from build123d import *

# Parameters (mm, degrees)
BOSS_EXTRUDE1_DEPTH      = 520.7
BOSS_EXTRUDE1_DEPTH_BACK = 520.7
SKETCH1_W                = 38.1
SKETCH1_H                = 25.4
SKETCH1_W_2              = 31.75
SKETCH1_H_2              = 19.05
SKETCH2_R                = 2.38125
CUT_EXTRUDE1_DEPTH       = 520.7
SKETCH3_R                = 2.38125
CUT_EXTRUDE2_DEPTH       = 100


with BuildPart() as part:
    # Sketch1 → Boss-Extrude1 (new, two sides: drawn at the far end of the back side and taken through both)
    with BuildSketch(Plane.XY.offset(-BOSS_EXTRUDE1_DEPTH_BACK)):
        Rectangle(SKETCH1_W, SKETCH1_H)
        Rectangle(SKETCH1_W_2, SKETCH1_H_2, mode=Mode.SUBTRACT)
    extrude(amount=BOSS_EXTRUDE1_DEPTH + BOSS_EXTRUDE1_DEPTH_BACK)

    # Sketch2 → Cut-Extrude1 (cut)
    with BuildSketch(Plane(origin=(0, 12.7, 0), x_dir=(1, 0, 0), z_dir=(0, 1, 0))):
        with Locations(Location((0, -384.81, 0), (0, 0, 180))):
            Circle(SKETCH2_R)
        with Locations(Location((0, -505.46, 0), (0, 0, 180))):
            Circle(SKETCH2_R)
    extrude(amount=-CUT_EXTRUDE1_DEPTH, mode=Mode.SUBTRACT)

    # Sketch3 → Cut-Extrude2 (cut)
    with BuildSketch(Plane(origin=(0, 12.7, 0), x_dir=(1, 0, 0), z_dir=(0, 1, 0))):
        with Locations(Location((0, 506.4125, 0), (0, 0, 180))):
            Circle(SKETCH3_R)
        with Locations(Location((0, 466.725, 0), (0, 0, 180))):
            Circle(SKETCH3_R)
    extrude(amount=-CUT_EXTRUDE2_DEPTH, mode=Mode.SUBTRACT)


solid = part.part
Source: CAD feature listing. Evaluate the final solid. Frame: model axes, mm. A direction names the side the tool comes from. Give positions to 0.01 mm unless a question says otherwise; leave off trailing zeros. Write each loop counter-clockwise with the first axis right and the second up, starting at its lowest first coordinate (ties: lowest second). Pieces come first, ordered by that corner, then holes. Notation, with made-up numbers: M -10,11 L -6,11 A8 cw -6,15 Z; hole C 51,68 d4. An arc over 180 degrees is marked long. Answer as a JSON object with one key per item and string values.
Q1. Cut plane A-A, the plane x = -8.5. Return the cut outline in (y, z) (3 decimals).
Geometry check:
{"outline": "M -12.7,-520.7 L -9.525,-520.7 L -9.525,520.7 L -12.7,520.7 Z; M 9.525,-520.7 L 12.7,-520.7 L 12.7,520.7 L 9.525,520.7 Z"}
Q2. Ray query, line 1 along Z through (x, y) = (0, 11.5); line 2 along X through (y, z) = (-1, -285) (3 decimals); line 3 along X through (y, z) = (-12, 505.46). Return the intervals inside material, ascending.
Geometry check:
{"line 1": "z = -520.7 to -508.79, -504.03 to -469.11, -464.34 to 382.43, 387.19 to 503.08, 507.84 to 520.7", "line 2": "x = -19.05 to -15.875, 15.875 to 19.05", "line 3": "x = -19.05 to -2.38, 2.38 to 19.05"}
Q3. Mould query, pull axis Y, two halves, no side actions, for faces 3 (the face through (0, 12.7, -7)), 4 (the face through (0, -9.525, -7)), 5 (the face through (0, -11, 520.7)). Classes: +Y half, -Y half, draft (parallel to the pull), parting line (faces both ways), or undercut.
Geometry check:
{"face 3": "+Y half", "face 4": "undercut", "face 5": "draft"}
Q4. Cut plane B-B, the plane z = -267.5. Return the cut outline in (x, y) (3 decimals), then the cut area to 3 significant figures.
Geometry check:
{"outline": "M -19.05,-12.7 L 19.05,-12.7 L 19.05,12.7 L -19.05,12.7 Z; hole M -15.875,-9.525 L 15.875,-9.525 L 15.875,9.525 L -15.875,9.525 Z", "area": "363 mm^2"}
Q5. Access query for faces 1 (the face through (-19.05, 0, -7)), 2 (the face through (15.875, 0, -7)). Directions: +Z, -Z, +X, -X, +Y, -Y. A direction counts if a zero-diameter tool reaches every point of the face in a straight line with its end or side. Return the directions, or none.
Geometry check:
{"face 1": "+Z, -Z, -X, +Y, -Y", "face 2": "+Z, -Z"}
Q6. Cut plane C-C, the plane y = 3.75. Return the cut outline in (x, z) (3 decimals).
Geometry check:
{"outline": "M -19.05,-520.7 L -15.875,-520.7 L -15.875,520.7 L -19.05,520.7 Z; M 15.875,-520.7 L 19.05,-520.7 L 19.05,520.7 L 15.875,520.7 Z"}
